Source: CAD feature listing. Evaluate the final solid. Frame: model axes, mm. Face numbers are marked on the shaded views. Round coordinates to 2 decimals unless told otherwise and drop trailing zeros. Loops run counter-clockwise (first coordinate to the right, second up) from the corner with the lowest first, then second, coordinate; pieces in that order, holes last.
Item 1: Section query B-B on y = -24.5. Return loops of the section in (x, z).
Item 2: First-contact query: P1, Ø2, axis at x = 73.5, z = 7.5, coming from the -Y side; P2, Ø1, axis at y = -17, z = 8.5, coming from the +X side; P3, Ø2, axis at y = -15, z = 6.5, coming from the -X side. Flat tips, straight axial feed; report the tip coordinate or a pass-through.
Item 3: Section query C-C on z = 7.5. Give the number of separate pieces and of enclosed holes in the cut face, then the cut area to 3 significant figures.
Item 4: Pull-direction query (X, two-part tool) for the marked faces 1, 2 and 3; classes: released by +X, released by -X, zero draft, split by the parting line, or undercut.
Item 5: Section query A-A on x = 27.5. Return loops of the section in (y, z).
Item 6: Section query D-D on x = 88. Return loops of the section in (y, z).
Item 7: Ray query, L1, parallel to X at y = -8, z = 8.25; L2, parallel to X at y = -48, z = 8.5; L3, parallel to Y at x = 12.5, z = 5.25. Return the intervals inside material, ascending.
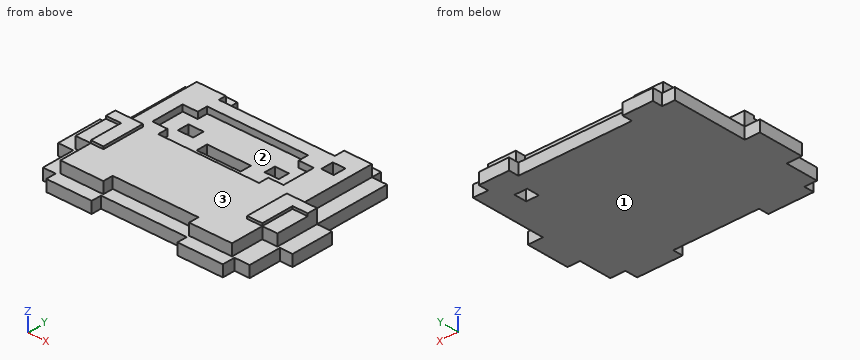
Autodesk Fusion 360 part; units mm, degrees
sketch "finn" plane through (0, 0, 0) normal (0, 0, 1) x (1, 0, 0)
  line L0 (12, 6) -> (12, -23)
  line L1 (12, -23) -> (6, -23)
  line L2 (6, -23) -> (6, -41)
  line L3 (6, -41) -> (12, -41)
  line L4 (12, -41) -> (12, -54)
  line L5 (12, -54) -> (17, -54)
  line L6 (17, -58) -> (35, -58)
  line L7 (35, -58) -> (35, -54)
  line L8 (35, -54) -> (69, -54)
  line L9 (69, -58) -> (87, -58)
  line L10 (87, -58) -> (87, -53)
  line L11 (87, -53) -> (93, -53)
  line L12 (93, -53) -> (93, -40)
  line L13 (98, -40) -> (98, -23)
  line L14 (98, -23) -> (92, -23)
  line L15 (92, -23) -> (92, 7)
  line L16 (92, 7) -> (86, 7)
  line L17 (86, 11) -> (74, 11)
  line L18 (74, 11) -> (74, 7)
  line L19 (74, 7) -> (29, 7)
  line L20 (29, 11) -> (17, 11)
  line L21 (17, 11) -> (17, 7)
  line L22 (12, 6) -> (12, 7)
  line L23 (23, -6) -> (23, -19)
  line L24 (23, -19) -> (29, -19)
  line L25 (29, -23) -> (69, -23)
  line L26 (69, -23) -> (69, -19)
  line L27 (75, -19) -> (75, -6)
  line L28 (75, -6) -> (69, -6)
  line L29 (69, -2) -> (69, -6)
  line L30 (69, -2) -> (29, -2)
  line L31 (29, -2) -> (29, -6)
  line L32 (23, -6) -> (29, -6)
  line L33 (29, -10.3517) -> (29, -14.5037)
  line L34 (29, -14.5037) -> (35, -14.5037)
  line L35 (35, -14.5037) -> (35, -10)
  line L36 (35, -10) -> (29, -10)
  line L37 (29, -10) -> (29, -10.3517)
  line L38 (63.4285, -10.1759) -> (69, -10.1759)
  line L39 (69, -10.1759) -> (69, -14.5392)
  line L40 (69, -14.5392) -> (63.393, -14.5392)
  line L41 (63.393, -14.5392) -> (63.4285, -10.1759)
  line L42 (40.5749, -14.5392) -> (40.5749, -19)
  line L43 (40.5749, -19) -> (58, -19)
  line L44 (58, -19) -> (58, -14.5392)
  line L45 (58, -14.5392) -> (40.5749, -14.5392)
  line L46 (17, -58) -> (17, -54)
  line L47 (29, 7) -> (29, 11)
  line L48 (12, 7) -> (17, 7)
  line L49 (12, -23) -> (12, -27)
  line L50 (12, -27) -> (18, -27)
  line L51 (18, -27) -> (18, -40)
  line L52 (18, -40) -> (23, -40)
  line L53 (23, -40) -> (23, -23)
  line L54 (23, -23) -> (12, -23)
  line L55 (92, -23) -> (80, -23)
  line L56 (80, -23) -> (80, -40)
  line L57 (80, -40) -> (86, -40)
  line L58 (86, -40) -> (86, -27)
  line L59 (86, -27) -> (92, -27)
  line L60 (92, -27) -> (92, -23)
  line L61 (69, -58) -> (69, -54)
  line L62 (12, -23) -> (12, -40)
  line L63 (12, -40) -> (18, -40)
  line L64 (18, -53) -> (35, -53)
  line L65 (35, -53) -> (35, -49)
  line L66 (35, -49) -> (69, -49)
  line L67 (69, -53) -> (69, -49)
  line L68 (69, -53) -> (86, -53)
  line L69 (86, -53) -> (86, -40)
  line L70 (86, -40) -> (92, -40)
  line L71 (92, -40) -> (92, -23)
  line L72 (92, -23) -> (86, -23)
  line L73 (92, -23) -> (86, -23)
  line L74 (86, -23) -> (86, 7)
  line L75 (86, 7) -> (75, 7)
  line L76 (75, 7) -> (75, 3)
  line L77 (75, 3) -> (29, 3)
  line L78 (29, 3) -> (29, 6)
  line L79 (29, 6) -> (17.5, 6)
  line L80 (17.5, 6) -> (17.5, -23)
  line L81 (18, -53) -> (18, -40)
  line L82 (93, -40) -> (98, -40)
  line L83 (86, 11) -> (86, 7)
  line L84 (29, -19) -> (29, -23)
  line L85 (69, -19) -> (75, -19)
  line L86 (23, -27) -> (80, -27)
  line L87 (23, -27) -> (23, -40)
extrude "Extrude7" add sketch "finn" along normal blind 10 contours L49 L50 L51 L52 L53 L54 L62 L87 | L55 L56 L57 L58 L59 L60 L71 L72 L73 makes body 1 at (23, -34.3333, 3.3333) makes body 2 at (80, -28.6667, 3.3333)
extrude "Extrude8" add sketch "finn" along normal blind 9 separate body contours L50 L51 L62 L63 | L53 L54 L55 L56 L74 L75 L76 L77 L78 L79 L80 L86 | L52 L53 L56 L57 L64 L65 L66 L67 L68 L69 L81 L86 L87 | L58 L59 L70 L71 makes body 3 at (44.3333, -31.6667, 0)
extrude "Extrude9" add sketch "finn" along normal blind 6.5 contours L23 L24 L25 L26 L27 L28 L29 L30 L31 L32 L84 L85 bodies 3
combine "Combine1" operation add target body 3 tool bodies 1 2
extrude "Extrude10" add sketch "finn" along normal blind 4.5 contours L0 L17 L18 L19 L20 L21 L22 L47 L48 L54 L75 L76 L77 L78 L79 L80 L83 | L1 L2 L3 L4 L5 L6 L7 L8 L9 L10 L11 L12 L13 L14 L46 L49 L60 L61 L62 L63 L64 L65 L66 L67 L68 L69 L70 L71 L81 L82 | L15 L16 L55 L72 L73 L74 bodies 3
extrude "Extrude11" add sketch "finn" along normal blind 2.5 contours L33 L34 L35 L36 L37 | L38 L39 L40 L41 | L42 L43 L44 L45 bodies 3
sketch "Sketch6" plane through (0, 0, 9) normal (0, 0, 1) x (-1, 0, 0)
  line L0 (-23, 19) -> (-23, 6)
  line L1 (-23, 6) -> (-29, 6)
  line L2 (-29, 6) -> (-29, 2)
  line L3 (-29, 2) -> (-69, 2)
  line L4 (-69, 2) -> (-69, 6)
  line L5 (-69, 6) -> (-75, 6)
  line L6 (-75, 6) -> (-75, 19)
  line L7 (-75, 19) -> (-69, 19)
  line L8 (-69, 19) -> (-69, 23)
  line L9 (-69, 23) -> (-29, 23)
  line L10 (-29, 23) -> (-29, 19)
  line L11 (-29, 19) -> (-23, 19)
  line L12 (-23, 23) -> (-23, 40)
  line L13 (-23, 40) -> (-18, 40)
  line L14 (-18, 40) -> (-18, 53)
  line L15 (-18, 53) -> (-35, 53)
  line L16 (-35, 53) -> (-35, 49)
  line L17 (-35, 49) -> (-69, 49)
  line L18 (-69, 49) -> (-69, 53)
  line L19 (-69, 53) -> (-86, 53)
  line L20 (-86, 53) -> (-86, 40)
  line L21 (-86, 40) -> (-80, 40)
  line L22 (-80, 40) -> (-80, 23)
  line L23 (-80, 23) -> (-86, 23)
  line L24 (-86, 23) -> (-86, -7)
  line L25 (-86, -7) -> (-75, -7)
  line L26 (-75, -7) -> (-75, -3)
  line L27 (-75, -3) -> (-29, -3)
  line L28 (-29, -3) -> (-29, -6)
  line L29 (-29, -6) -> (-17.5, -6)
  line L30 (-17.5, -6) -> (-17.5, 23)
  line L31 (-17.5, 23) -> (-23, 23)
  line L32 (-77, 0) -> (-82, 0)
  line L33 (-82, 0) -> (-82, 5)
  line L34 (-82, 5) -> (-77, 5)
  line L35 (-77, 5) -> (-77, 0)
extrude "Extrude13" cut sketch "Sketch6" against normal blind 10 contours L32 L33 L34 L35 bodies 3
Data:
1. outline: (6, 0) - (98, 0) - (98, 4.5) - (92, 4.5) - (92, 10) - (80, 10) - (80, 9) - (23, 9) - (23, 10) - (12, 10) - (12, 4.5) - (6, 4.5) - close
2. P1: stops at y = -53
2. P2: stops at x = 86
2. P3: stops at x = 17.5
3. separate pieces: 1
3. enclosed holes: 2
3. area: 2,950 mm2
4. face 1: zero draft
4. face 2: undercut
4. face 3: undercut
5. outline: (-58, 0) - (11, 0) - (11, 4.5) - (6, 4.5) - (6, 9) - (-6, 9) - (-6, 6.5) - (-19, 6.5) - (-19, 9) - (-53, 9) - (-53, 4.5) - (-58, 4.5) - close
6. outline: (-53, 0) - (7, 0) - (7, 4.5) - (-23, 4.5) - (-23, 10) - (-27, 10) - (-27, 9) - (-40, 9) - (-40, 4.5) - (-53, 4.5) - close
7. L1: x = 17.5 to 23, 75 to 86
7. L2: x = 18 to 86
7. L3: y = -40 to -23
